Input: part model. Units: mm. Frame: model coordinates. Coordinates: 2 decimals unless noted, no trailing zeros. Order: outer loops, then holes, each group sorted by start corner. A loop starts at its lowest first (then second) coordinate and runs counter-clockwise, first axis right, second up. Notation, with made-up numbers: (71, -15.75) -> (113, -15.75) arc R21 cw to (113, 1.25) -> close; hole circle Ø3 at (63.5, 48.5). An arc over 180 degrees is marked (long way). Write each question's results on one line, items separated by ' | '.
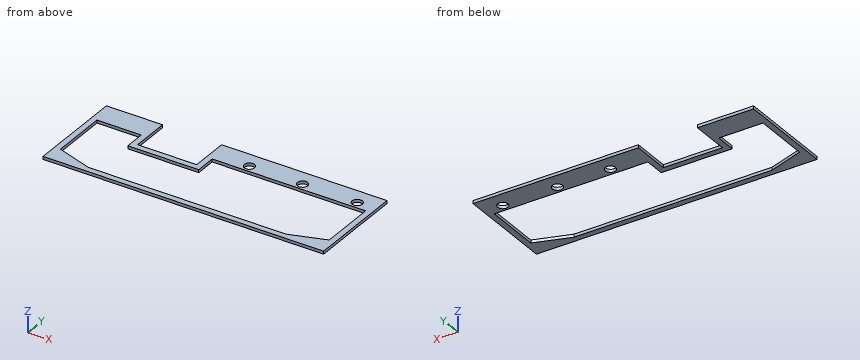
```python
from build123d import *

# Parameters (mm, degrees)
BOSS_EXTRUDE2_DEPTH   = 1
CUT_EXTRUDE2_DEPTH    = 1
F_3_0MM_DOWEL_HOLE1_D = 3.5


with BuildPart() as part:
    # Sketch2 → Boss-Extrude2 (new body)
    with BuildSketch(Plane.XY):
        Polygon((2, 8), (2, -25), (-93, -25), (-93, 8), (-74, 8), (-74, -5), (-54, -5), (-54, 8), align=None)
    extrude(amount=BOSS_EXTRUDE2_DEPTH)

    # Sketch1 → Cut-Extrude2 (cut)
    with BuildSketch(Plane.XY):
        Polygon((0, 0), (0, -19), (-12, -23), (-79, -23), (-91, -19), (-91, 0), (-76, 0), (-76, -7), (-52, -7), (-52, 0), align=None)
    extrude(amount=CUT_EXTRUDE2_DEPTH, mode=Mode.SUBTRACT)

    # Ø3.0mm Dowel Hole1 (through all)
    with Locations(Plane.XY.offset(1)):
        with Locations((-41, 2.5), (-23, 2.5), (-4.5, 2.5)):
            Hole(F_3_0MM_DOWEL_HOLE1_D / 2)


solid = part.part
```
(1) Line query: line 1 along Y through (x, z) = (-23, 0.65); line 2 along Y through (x, z) = (-46.5, 0.7); line 3 along X through (y, z) = (-12, 0.55). Output: solid intervals per line, ascending. Write a range as from..to.
Return value:
line 1: -25..-23, 0..0.75, 4.25..8 | line 2: -25..-23, 0..8 | line 3: -93..-91, 0..2
(2) Cut plane B-B, the plane z = 0.3. Return loops of the section in (x, y), plus the area to 3 significant figures.
Return value:
outline: (-93, -25) -> (2, -25) -> (2, 8) -> (-54, 8) -> (-54, -5) -> (-74, -5) -> (-74, 8) -> (-93, 8) -> close; hole (-91, -19) -> (-79, -23) -> (-12, -23) -> (0, -19) -> (0, 0) -> (-52, 0) -> (-52, -7) -> (-76, -7) -> (-76, 0) -> (-91, 0) -> close; hole circle Ø3.5 at (-41, 2.5); hole circle Ø3.5 at (-23, 2.5); hole circle Ø3.5 at (-4.5, 2.5) | area: 969 mm2
(3) Cut plane C-C, the plane y = 2.5. Return loops of the section in (x, z).
Return value:
outline: (-93, 0) -> (-74, 0) -> (-74, 1) -> (-93, 1) -> close; (-54, 0) -> (-42.75, 0) -> (-42.75, 1) -> (-54, 1) -> close; (-39.25, 0) -> (-24.75, 0) -> (-24.75, 1) -> (-39.25, 1) -> close; (-21.25, 0) -> (-6.25, 0) -> (-6.25, 1) -> (-21.25, 1) -> close; (-2.75, 0) -> (2, 0) -> (2, 1) -> (-2.75, 1) -> close
(4) Cut plane A-A, the plane x = -23. Return loops of the section in (y, z).
Return value:
outline: (-25, 0) -> (-23, 0) -> (-23, 1) -> (-25, 1) -> close; (0, 0) -> (0.75, 0) -> (0.75, 1) -> (0, 1) -> close; (4.25, 0) -> (8, 0) -> (8, 1) -> (4.25, 1) -> close
(5) Cut plane D-D, the plane x = -67. Return loops of the section in (y, z), plus the area to 3 significant figures.
Return value:
outline: (-25, 0) -> (-23, 0) -> (-23, 1) -> (-25, 1) -> close; (-7, 0) -> (-5, 0) -> (-5, 1) -> (-7, 1) -> close | area: 4.00 mm2
